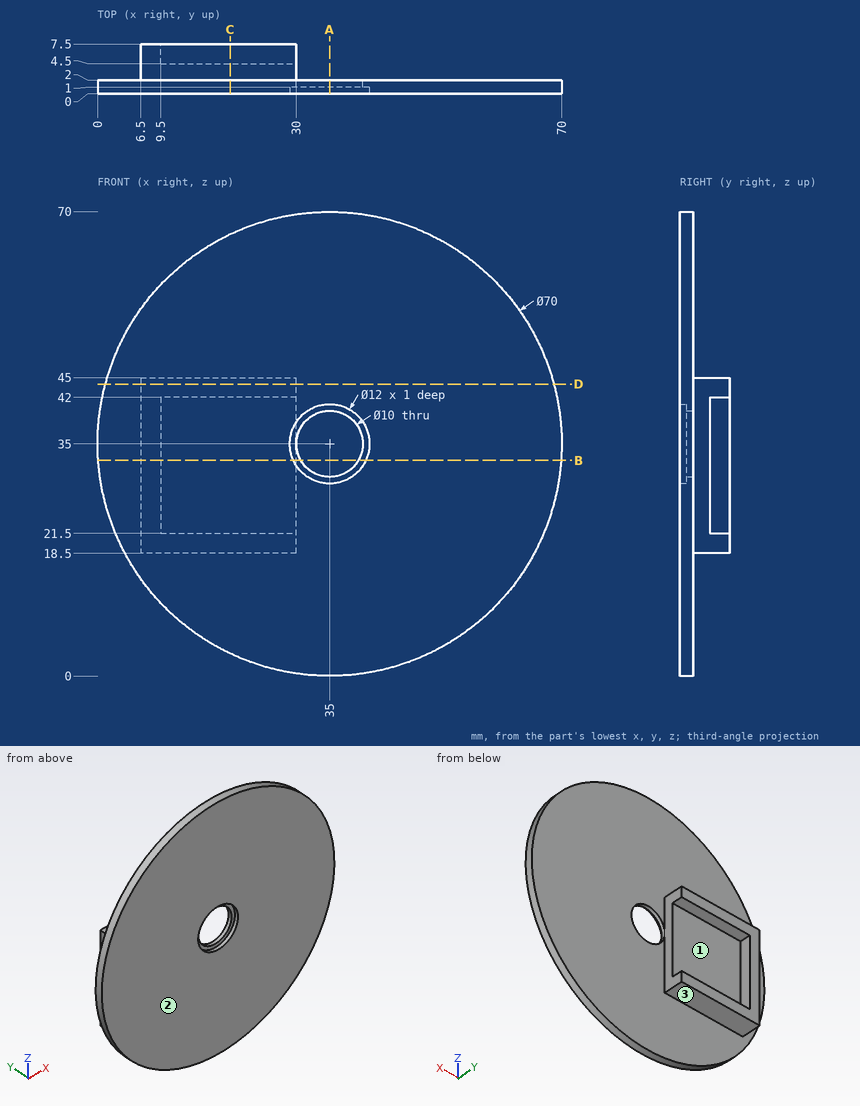
Source: three-view drawing plus pictorial views. Frame: mm from the lowest corner of the part. Coordinates: 2 decimals unless noted, no trailing zeros. Loops run counter-clockwise (first coordinate to the right, second up) from the corner with the lowest first, then second, coordinate; pieces in that order, holes last. Notation, with made-up numbers: M -4,-13.5 L 22,-13.5 A9 ccw 22,-9.5 Z; hole C 6,-10.5 d2. An arc over 180 degrees is marked long. Use CSV: the item, a comma, the result in double quotes.
(1) Line query: line 1 (X direction, y = 1.25, z = 35); line 2 (X direction, y = 0.65, z = 35); line 3 (Y direction, x = 60, z = 33.5). Output: solid intervals per line, ascending. Write a range as [from, to].
Answers follow:
line 1,"[0, 30], [40, 70]"
line 2,"[0, 29], [41, 70]"
line 3,"[0, 2]"
(2) Cut plane D-D on z = 44. Return loops of the section in (x, y), and give its area (3 significant figures).
Answers follow:
outline,"M 1.18,0 L 68.82,0 L 68.82,2 L 30,2 L 30,7.5 L 6.5,7.5 L 6.5,2 L 1.18,2 Z"
area,"265 mm²"
(3) Cut plane B-B on z = 32.5. Return loops of the section in (x, y), and give its area (3 significant figures).
Answers follow:
outline,"M 0.09,0 L 29.55,0 L 29.55,1 L 30.67,1 L 30.67,2 L 30,2 L 30,4.5 L 9.5,4.5 L 9.5,7.5 L 6.5,7.5 L 6.5,2 L 0.09,2 Z; M 39.33,1 L 40.45,1 L 40.45,0 L 69.91,0 L 69.91,2 L 39.33,2 Z"
area,"188 mm²"
(4) Draft query along Z for the marked faces 1, 2 and 3. Return one class per face: pulls with the +Z half, pulls with the -Z half, needs draft (parallel to the pull), parting line crosses it, or undercut.
Answers follow:
face 1,"undercut"
face 2,"needs draft"
face 3,"pulls with the -Z half"
(5) Cut plane C-C on x = 20. Return loops of the section in (y, z).
Answers follow:
outline,"M 0,3.38 L 2,3.38 L 2,18.5 L 7.5,18.5 L 7.5,21.5 L 4.5,21.5 L 4.5,42 L 7.5,42 L 7.5,45 L 2,45 L 2,66.62 L 0,66.62 Z"
(6) Contact query for flat-ended pins moving along their axis: pin 1 (0.9 mm diameter, centred on x = 16.5, y = 6.5, fed in from -Z); pin 2 (10 mm diameter, centred on x = 16, z = 27.5, fed in from +Y); pin 3 (1.6 mm diameter, centred on y = 3.5, z = 33, fed in from -X); pin 4 (10 mm diameter, centred on x = 52, z = 24.5, fed in from -Y). Output: stop coordinate, or through.
Answers follow:
pin 1,"z = 18.5"
pin 2,"y = 4.5"
pin 3,"x = 6.5"
pin 4,"y = 0"
(7) Cut plane A-A on x = 35. Return loops of the section in (y, z).
Answers follow:
outline,"M 0,0 L 2,0 L 2,30 L 1,30 L 1,29 L 0,29 Z; M 0,41 L 1,41 L 1,40 L 2,40 L 2,70 L 0,70 Z"
